The model under review builds one solid part; all positions refer to its coordinate system, in mm. Face numbers are marked on the shaded views. Coordinates: 2 decimals unless noted, no trailing zeros. Order: outer loops, then holes, each group sorted by start corner. A loop starts at its lowest first (then second) coordinate and runs counter-clockwise, first axis right, second up. Notation, with made-up numbers: (88, 86.5) -> (92, 86.5) arc R6 cw to (92, 97.5) -> close; hole circle Ø4 at (-38.75, 7.25). An arc over 180 degrees is marked (long way). Use one line per item in the form item = value. Start each with the question number.
(1) Take a section at A-A (x = 0). State the section outline as (y, z) points, then the cut area to 3 significant figures.
(2) Insertion check: pin 1 Ø8 at (x, y) = (2.5, 0.5) entering from -Z; pin 2 Ø8 at (y, z) = (-6, 90.5) entering from +X. Each pin has a flat end and moves straight along its axis. Give the tip position at first contact, or say it passes through.
(3) Wall thickness on line 1 along Y through (x, z) = (0, 94); line 2 along X through (y, z) = (-3.25, 66); line 3 along Y through (x, z) = (-3.75, 97.5): over which ranges is each line inside the solid? List them lowest first.
(4) Mouldability with a two-part tool opening along Y and no side actions: class the marked faces 1 and 2 as +Y half, -Y half, draft (parallel to the pull), parting line (faces both ways), or undercut.
(5) Take a section at C-C (z = 101). State the section outline as (x, y) points (1 decimal), then the cut area to 3 significant figures.
```python
from build123d import *

# Parameters (mm, degrees)
EXTRUDE1_DEPTH  = 58.42
SKETCH2_R       = 7.62
EXTRUDE2_DEPTH  = 50
SKETCH3_R       = 6.0325
EXTRUDE12_DEPTH = 110.253593305
FILLET1_R       = 0.762


with BuildPart() as part:
    # Sketch1 → Extrude1 (new body)
    with BuildSketch(Plane.XY):
        with BuildLine():
            Line((-9.525, 8.699334611), (9.525, 8.699334611))
            Line((9.525, 8.699334611), (9.525, 0))
            ThreePointArc((9.525, 0), (0, -9.525), (-9.525, 0))
            Line((-9.525, 0), (-9.525, 8.699334611))
        make_face()
    extrude(amount=EXTRUDE1_DEPTH)


with BuildPart() as body_2:
    # Sketch2 → Extrude2 (new body)
    with BuildSketch(Plane.XY.offset(58.42)):
        Circle(SKETCH2_R)
    extrude(amount=EXTRUDE2_DEPTH)


with BuildPart() as extrude12_tool:
    # Sketch3 → Extrude12 (new, through all)
    with BuildSketch(Plane.XY.offset(108.42)):
        Circle(SKETCH3_R)
    extrude(amount=-EXTRUDE12_DEPTH)


with BuildPart() as part_1:
    add(part.part)

    # Extrude12: cut by extrude12_tool
    add(extrude12_tool.part, mode=Mode.SUBTRACT)


with BuildPart() as body_2_1:
    add(body_2.part)

    # Extrude12: cut by extrude12_tool
    add(extrude12_tool.part, mode=Mode.SUBTRACT)

    # Fillet1
    fillet1_edges = [body_2_1.edges().sort_by_distance(p)[0] for p in [
        (-7.62, 0, 108.42),
    ]]
    fillet(fillet1_edges, radius=FILLET1_R)


solid = body_2_1.part
```
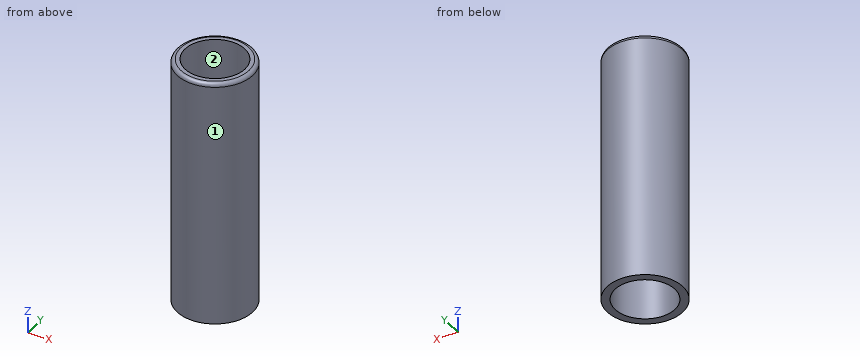
Findings:
q1.outline = (-7.62, 58.42) -> (-6.03, 58.42) -> (-6.03, 108.42) -> (-6.86, 108.42) arc R0.76 ccw to (-7.62, 107.66) -> close; (6.03, 58.42) -> (7.62, 58.42) -> (7.62, 107.66) arc R0.76 ccw to (6.86, 108.42) -> (6.03, 108.42) -> close
q1.area = 159 mm²
q2.pin_1 = 58.42
q2.pin_2 = 7.35
q3.line_1 = -7.62 to -6.03, 6.03 to 7.62
q3.line_2 = -6.89 to -5.08, 5.08 to 6.89
q3.line_3 = -6.63 to -4.73, 4.73 to 6.63
q4.face_1 = parting line
q4.face_2 = undercut
q5.outline = circle Ø15.2 at (0, 0); hole circle Ø12.1 at (0, 0)
q5.area = 68.1 mm²
